```python
from build123d import *

# Parameters (mm, degrees)
F0_W          = 72
F0_H          = 30
F1_DEPTH      = 62
F3_DEPTH      = 30.001
F4_W          = 15
F4_H          = 47
F5_DEPTH      = 36.001
F5_DEPTH_BACK = 25
F6_W          = 20
F6_H          = 10
F7_DEPTH      = 62.001
F9_D          = 9
F10_R         = 3
F11_R         = 3
F12_R         = 3
F13_R         = 2


with BuildPart() as f1:
    # F0 (on Top) → F1 (new body)
    with BuildSketch(Plane.XY):
        Rectangle(F0_W, F0_H)
    extrude(amount=F1_DEPTH)

    # F2 (on face) → F3 (cut, through all)
    with BuildSketch(Plane.XZ.offset(15)):
        Polygon((-15, 72), (-46, 72), (-46, 20), (-20, 20), (-15, 62), align=None)
        Polygon((46, 72), (15, 72), (15, 62), (20, 20), (46, 20), align=None)
    extrude(amount=-F3_DEPTH, mode=Mode.SUBTRACT)

    # F4 (on Right) → F5 (cut, two sides)
    with BuildSketch(Plane.YZ) as f5_sk:
        with Locations((-17.5, 48.5)):
            Rectangle(F4_W, F4_H)
        with Locations((17.5, 48.5)):
            Rectangle(F4_W, F4_H)
    extrude(amount=-F5_DEPTH, mode=Mode.SUBTRACT)
    extrude(f5_sk.sketch, amount=F5_DEPTH_BACK, mode=Mode.SUBTRACT)

    # F6 (on face) → F7 (cut, through all)
    with BuildSketch(Plane.XY.offset(62)):
        Rectangle(F6_W, F6_H)
    extrude(amount=-F7_DEPTH, mode=Mode.SUBTRACT)

    # F9 (through all)
    with Locations(Plane.XY.offset(20)):
        with Locations((-28, 0), (28, 0)):
            Hole(F9_D / 2)

    # F10
    f10_edges = [f1.edges().sort_by_distance(p)[0] for p in [
        (-36, 15, 10),
        (36, -15, 10),
        (36, 15, 10),
        (-36, -15, 10),
    ]]
    fillet(f10_edges, radius=F10_R)

    # F11
    f11_edges = [f1.edges().sort_by_distance(p)[0] for p in [
        (-20, 0, 20),
        (20, 0, 20),
    ]]
    fillet(f11_edges, radius=F11_R)

    # F12
    f12_edges = [f1.edges().sort_by_distance(p)[0] for p in [
        (0, 10, 25),
        (0, -10, 25),
    ]]
    fillet(f12_edges, radius=F12_R)

    # F13
    f13_edges = [f1.edges().sort_by_distance(p)[0] for p in [
        (10, 5, 31),
        (10, -5, 31),
        (-10, -5, 31),
        (-10, 5, 31),
    ]]
    fillet(f13_edges, radius=F13_R)


solid = f1.part
```
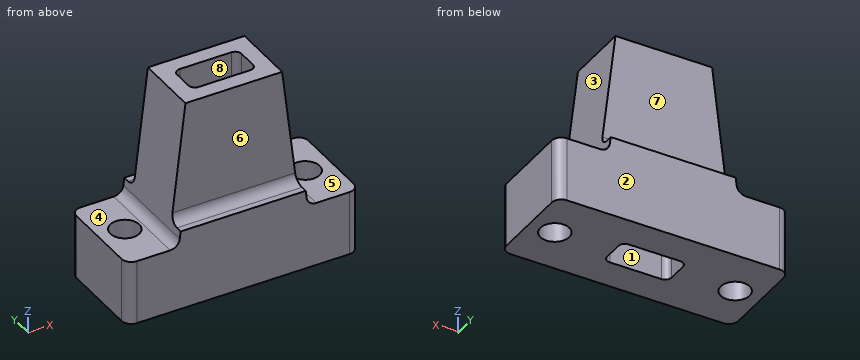
Work out the finished part from the listing and answer in its coordinate system (mm). Face numbers are marked on the shaded views. A direction names the side the tool comes from. Round coordinates to 2 decimals unless told otherwise and drop trailing zeros. Write each loop counter-clockwise with the first axis right and the second up, starting at its lowest first coordinate (ties: lowest second). Pieces come first, ordered by that corner, then holes. Notation, with made-up numbers: (33, -20.5) - (72, -20.5) arc R11 ccw to (72, -6.5) - close; hole circle Ø8 at (66.5, 19). An arc over 180 degrees is marked (long way). Return JSON: item names as keys, results as strings. Group by question number.
Q1. For the marked faces 4, 5, 6, 7 and 8, determine the directions among +Z, -Z, +X, -X, +Y, -Y from which every point of the face is accessible in a straight line to the end or side of a thin tool.
Q2. Each of these flat-tipped pins is pushed along its axis until it touches: pin 1 Ø10.5 at (x, y) = (-31.5, -5) entering from +Z; pin 2 Ø17.5 at (x, z) = (1.5, 25.5) entering from -Y; pin 3 Ø5 at (y, z) = (0.5, 45.5) entering from +X; pin 4 Ø1 at (x, y) = (-3.5, 13.5) entering from +Z. Where does it stop, or does it pass through?
Q3. Find the intervals of material crossed by L1, parallel to Y at x = -28, z = 9; L2, parallel to Y at x = 2, z = 37; L3, parallel to Z at x = 8.5, y = -13, in increasing order.
Q4. The mould has two halves that part along Y. Classify the marked faces 1, 2 and 3: released by +Y, released by -Y, zero draft, split by the parting line, or undercut.
Q5. The part is cut by section A-A on x = 28. Write down the section's boundary in (y, z).
Q6. The part is cut by section D-D on y = 0. Write down the section's boundary in (x, z), then the cut area to 3 significant figures.
Q7. The part is cut by section B-B on y = 8. Write down the section's boundary in (x, z), then the cut area to 3 significant figures.
Q8. The part is cut by section C-C on z = 16. Write down the section's boundary in (x, y), then the cut area to 3 significant figures.
Solved:
{
 "1": {"face 4": "+Z, -X, +Y, -Y", "face 5": "+Z, +X, +Y, -Y", "face 6": "+Z, +X, -X, -Y", "face 7": "+Z, +X, -X, +Y", "face 8": "+Z, -Z"},
 "2": {"pin 1": "z = 20", "pin 2": "y = -15", "pin 3": "x = 17.26", "pin 4": "z = 25"},
 "3": {"L1": "-15 to -4.5, 4.5 to 15", "L2": "-10 to -5, 5 to 10", "L3": "0 to 25"},
 "4": {"face 1": "undercut", "face 2": "released by +Y", "face 3": "zero draft"},
 "5": {"outline": "(-15, 0) - (-4.5, 0) - (-4.5, 20) - (-15, 20) - close; (4.5, 0) - (15, 0) - (15, 20) - (4.5, 20) - close"},
 "6": {"outline": "(-36, 0) - (-32.5, 0) - (-32.5, 20) - (-36, 20) - close; (-23.5, 0) - (-10, 0) - (-10, 62) - (-15, 62) - (-19.69, 22.65) arc R3 cw to (-22.66, 20) - (-23.5, 20) - close; (10, 0) - (23.5, 0) - (23.5, 20) - (22.66, 20) arc R3 cw to (19.69, 22.65) - (15, 62) - (10, 62) - close; (32.5, 0) - (36, 0) - (36, 20) - (32.5, 20) - close", "area": "1,310 mm²"},
 "7": {"outline": "(-36, 0) - (36, 0) - (36, 20) - (22.66, 20) arc R3 cw to (19.69, 22.65) - (15, 62) - (-15, 62) - (-19.69, 22.65) arc R3 cw to (-22.66, 20) - (-36, 20) - close", "area": "2,910 mm²"},
 "8": {"outline": "(-36, -12) arc R3 ccw to (-33, -15) - (33, -15) arc R3 ccw to (36, -12) - (36, 12) arc R3 ccw to (33, 15) - (-33, 15) arc R3 ccw to (-36, 12) - close; hole circle Ø9 at (-28, 0); hole (-10, -3) arc R2 ccw to (-8, -5) - (8, -5) arc R2 ccw to (10, -3) - (10, 3) arc R2 ccw to (8, 5) - (-8, 5) arc R2 ccw to (-10, 3) - close; hole circle Ø9 at (28, 0)", "area": "1,830 mm²"}
}
